For this review, take the finished solid that the model builds, in its own axes (mm). Coordinates: 2 decimals unless noted, no trailing zeros. Loops run counter-clockwise (first coordinate to the right, second up) from the corner with the lowest first, then second, coordinate; pieces in that order, holes last. Notation, with made-up numbers: (-27, -1) - (21, -1) arc R35 ccw to (21, 34) - close; hole circle Ø2 at (34, -34). An arc over 180 degrees is marked (long way). One line per item, written item: value. Start each with the question number.
1. Insertion check: pin 1 (1.5 mm diameter, centred on x = 250.5, y = 1, fed in from +Z); pin 2 (1 mm diameter, centred on x = 57.5, y = 1.5, fed in from +Z); pin 3 (2.5 mm diameter, centred on x = 0, z = -54, fed in from +Y); pin 4 (1.5 mm diameter, centred on x = 7.5, y = 1.5, fed in from +Z). Each pin has a flat end and moves straight along its axis. Give the tip position at first contact, or say it passes through.
2. Take a section at B-B, the plane x = -23. State the section outline as (y, z) points, and give its area (3 significant figures).
3. Take a section at C-C, the plane y = 2.1. Count the separate pieces of the cut face and the enclosed holes in it, and give its area (3 significant figures).
4. To check wall thickness, follow line 1 (Z direction, x = 248.5, y = 1.4); line 2 (Z direction, x = -27.5, y = 0.85); line 3 (X direction, y = 0.9, z = 37.5). State the ranges of each line that lie inside material, in increasing order. Write a range as from..to.
5. Take a section at D-D, the plane x = 259. State the section outline as (y, z) points, and give its area (3 significant figures).
6. Take a section at A-A, the plane z = 25.5. State the section outline as (x, y) points.
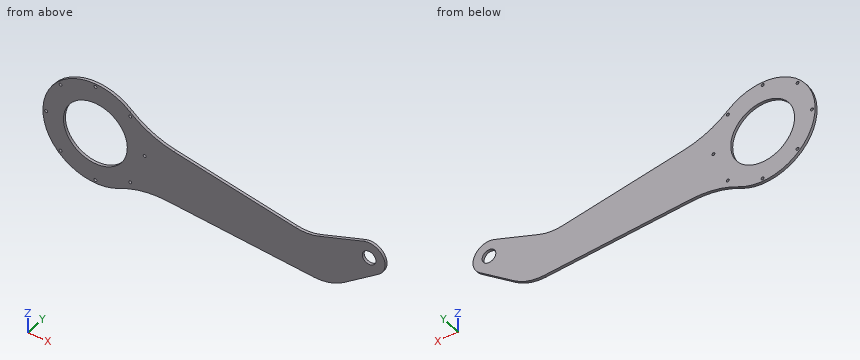
```python
from build123d import *

# Parameters (mm, degrees)
SKETCH1_R           = 1.6
SKETCH1_R_2         = 35
SKETCH1_R_3         = 7.5
BOSS_EXTRUDE2_DEPTH = 3
FILLET1_R           = 50
FILLET2_R           = 100


with BuildPart() as part:
    # Sketch1 → Boss-Extrude2 (new body)
    with BuildSketch(Plane(origin=(0, 0, 0), x_dir=(1, 0, 0), z_dir=(0, 1, 0))):
        with BuildLine():
            Line((257.543524338, 52.623283), (43.136797408, 38.01929391))
            ThreePointArc((43.136797408, 38.01929391), (-57.072915612, -6.99516287), (51.041719813, -26.476269347))
            Line((51.041719813, -26.476269347), (232.634460204, 5.800541986))
            Line((232.634460204, 5.800541986), (294.037229007, -16.452822314))
            ThreePointArc((294.037229007, -16.452822314), (315.449808374, -8.21908883), (310.311776158, 14.139210461))
            Line((310.311776158, 14.139210461), (257.543524338, 52.623283))
        make_face()
        with Locations(Location((38.183766184, 38.183766184, 0), (0, 0, 270))):
            Circle(SKETCH1_R, mode=Mode.SUBTRACT)
        with Locations(Location((0, 0, 0), (0, 0, 270))):
            Circle(SKETCH1_R_2, mode=Mode.SUBTRACT)
        with Locations(Location((54, 0, 0), (0, 0, 270))):
            Circle(SKETCH1_R, mode=Mode.SUBTRACT)
        with Locations(Location((0, 54, 0), (0, 0, 270))):
            Circle(SKETCH1_R, mode=Mode.SUBTRACT)
        with Locations(Location((-38.183766184, 38.183766184, 0), (0, 0, 270))):
            Circle(SKETCH1_R, mode=Mode.SUBTRACT)
        with Locations(Location((-54, 0, 0), (0, 0, 270))):
            Circle(SKETCH1_R, mode=Mode.SUBTRACT)
        with Locations(Location((0, -54, 0), (0, 0, 270))):
            Circle(SKETCH1_R, mode=Mode.SUBTRACT)
        with Locations(Location((-38.183766184, -38.183766184, 0), (0, 0, 270))):
            Circle(SKETCH1_R, mode=Mode.SUBTRACT)
        with Locations(Location((38.183766184, -38.183766184, 0), (0, 0, 270))):
            Circle(SKETCH1_R, mode=Mode.SUBTRACT)
        with Locations(Location((300, 0, 0), (0, 0, 270))):
            Circle(SKETCH1_R_3, mode=Mode.SUBTRACT)
    extrude(amount=BOSS_EXTRUDE2_DEPTH)

    # Fillet1
    fillet1_edges = [part.edges().sort_by_distance(p)[0] for p in [
        (232.634460204, 1.5, -5.800541986),
        (257.543524338, 1.5, -52.623283),
    ]]
    fillet(fillet1_edges, radius=FILLET1_R)

    # Fillet2
    fillet2_edges = [part.edges().sort_by_distance(p)[0] for p in [
        (51.041719813, 1.5, 26.476269347),
        (43.136797408, 1.5, -38.01929391),
    ]]
    fillet(fillet2_edges, radius=FILLET2_R)


solid = part.part
```
Solutions:
1. pin 1: z = 0.95
1. pin 2: z = 30.19
1. pin 3: through
1. pin 4: z = 57.1
2. outline: (0, -52.7) - (3, -52.7) - (3, -26.38) - (0, -26.38) - close; (0, 26.38) - (3, 26.38) - (3, 52.7) - (0, 52.7) - close
2. area: 158 mm2
3. separate pieces: 1
3. enclosed holes: 10
3. area: 20,100 mm2
4. line 1: -51.17..-0.05
4. line 2: -50.5..-21.65, 21.65..50.5
4. line 3: -43.59..-39.63, -36.74..36.74, 39.63..45.16
5. outline: (0, -48.8) - (3, -48.8) - (3, 3.75) - (0, 3.75) - close
5. area: 158 mm2
6. outline: (-51.54, 0) - (-23.97, 0) - (-23.97, 3) - (-51.54, 3) - close; (23.97, 0) - (67.3, 0) - (67.3, 3) - (23.97, 3) - close
